Check sheet for the modelled part. Datum: model origin and axes. Units: mm. A direction names the side the tool comes from. Coordinates: 2 decimals unless noted, no trailing zeros. Loops run counter-clockwise (first coordinate to the right, second up) from the corner with the lowest first, then second, coordinate; pieces in that order, holes last. Notation, with made-up numbers: M -37,66 L -31,66 A19 cw -31,80 Z; hole C -11.75,45.5 d5. An arc over 180 degrees is marked long. Write each question's results on one line, items separated by ' | '. Start each with the question number.
from build123d import *

# Parameters (mm, degrees)
SKETCH1_W                      = 96
SKETCH1_H                      = 96
BOSS_EXTRUDE1_DEPTH            = 8
SKETCH2_W                      = 92
SKETCH2_H                      = 92
COMPONENT_PLATFORM_DEPTH       = 6
CABLE_SLOTS_DEPTH              = 6
INNER_CORNER_FILLETS_R         = 3
M3X0_5_TAPPED_HOLE1_AT_2_COUNT = 2
M3X0_5_TAPPED_HOLE1_AT_2_PITCH = 70
M3X0_5_TAPPED_HOLE2_AT_2_COUNT = 2
M3X0_5_TAPPED_HOLE2_AT_2_PITCH = 70
M1_4X0_3_TAPPED_HOLE1_D        = 1.1
M1_4X0_3_TAPPED_HOLE1_DEPTH    = 3.7
M1_4X0_3_TAPPED_HOLE1_TIP      = 0.33047334
SKETCH29_R                     = 12
HDD_EXTRUSION_CUTOUT_DEPTH     = 10
HDD_EXTRUSION_CUTOUT_2_DEPTH   = 10
M3X0_5_TAPPED_HOLE3_D          = 2.5
M3X0_5_TAPPED_HOLE3_DEPTH      = 10
M3X0_5_TAPPED_HOLE3_TIP        = 0.751075774


with BuildPart() as part:
    # Sketch1 → Boss-Extrude1 (new body)
    with BuildSketch(Plane.XY):
        Rectangle(SKETCH1_W, SKETCH1_H)
    extrude(amount=BOSS_EXTRUDE1_DEPTH)

    # Sketch2 → Component Platform (cut)
    with BuildSketch(Plane.XY.offset(8)):
        Rectangle(SKETCH2_W, SKETCH2_H)
    extrude(amount=-COMPONENT_PLATFORM_DEPTH, mode=Mode.SUBTRACT)

    # Sketch3 → Cable Slots (cut, symmetric)
    with BuildSketch(Plane.XY.offset(2)):
        with BuildLine():
            Line((-33.878679656, -25.121320344), (-28.878679656, -20.121320344))
            ThreePointArc((-28.878679656, -20.121320344), (-28.228361402, -19.148050297), (-28, -18))
            Line((-28, -18), (-28, 18))
            ThreePointArc((-28, 18), (-28.228361402, 19.148050297), (-28.878679656, 20.121320344))
            Line((-28.878679656, 20.121320344), (-33.878679656, 25.121320344))
            ThreePointArc((-33.878679656, 25.121320344), (-34.851949703, 25.771638598), (-36, 26))
            Line((-36, 26), (-48, 26))
            Line((-48, 26), (-48, -26))
            Line((-48, -26), (-36, -26))
            ThreePointArc((-36, -26), (-34.851949703, -25.771638598), (-33.878679656, -25.121320344))
        make_face()
        with BuildLine():
            Line((48, -26), (48, 26))
            Line((48, 26), (36, 26))
            ThreePointArc((36, 26), (34.851949703, 25.771638598), (33.878679656, 25.121320344))
            Line((33.878679656, 25.121320344), (28.878679656, 20.121320344))
            ThreePointArc((28.878679656, 20.121320344), (28.228361402, 19.148050297), (28, 18))
            Line((28, 18), (28, -18))
            ThreePointArc((28, -18), (28.228361402, -19.148050297), (28.878679656, -20.121320344))
            Line((28.878679656, -20.121320344), (33.878679656, -25.121320344))
            ThreePointArc((33.878679656, -25.121320344), (34.851949703, -25.771638598), (36, -26))
            Line((36, -26), (48, -26))
        make_face()
    extrude(amount=CABLE_SLOTS_DEPTH, both=True, mode=Mode.SUBTRACT)

    # Inner Corner Fillets
    inner_corner_fillets_edges = [part.edges().sort_by_distance(p)[0] for p in [
        (-46, -46, 5),
        (-46, 46, 5),
        (46, 46, 5),
        (46, -46, 5),
    ]]
    fillet(inner_corner_fillets_edges, radius=INNER_CORNER_FILLETS_R)

    # Sketch14 → M3x0.5 Tapped Hole1 (revolve, cut)
    with BuildSketch(Plane(origin=(48, -35, 5), x_dir=(0, 0, -1), z_dir=(0, 1, 0))):
        Polygon((0, 0), (0, 10.751075774), (1.25, 10), (1.25, 0), align=None)
    m3x0_5_tapped_hole1 = revolve(axis=Axis((54.35, -35, 5), (-1, 0, 0)), mode=Mode.SUBTRACT)

    # M3x0.5 Tapped Hole1 at 2: M3x0.5 Tapped Hole1 ×2
    with Locations(*[(0, i * M3X0_5_TAPPED_HOLE1_AT_2_PITCH, 0) for i in range(1, M3X0_5_TAPPED_HOLE1_AT_2_COUNT)]):
        add(m3x0_5_tapped_hole1, mode=Mode.SUBTRACT)

    # Sketch16 → M3x0.5 Tapped Hole2 (revolve, cut)
    with BuildSketch(Plane(origin=(35, 48, 5), x_dir=(0, 0, 1), z_dir=(1, 0, 0))):
        Polygon((0, 0), (0, 10.751075774), (1.25, 10), (1.25, 0), align=None)
    m3x0_5_tapped_hole2 = revolve(axis=Axis((35, 54.35, 5), (0, -1, 0)), mode=Mode.SUBTRACT)

    # M3x0.5 Tapped Hole2 at 2: M3x0.5 Tapped Hole2 ×2
    with Locations(*[(-i * M3X0_5_TAPPED_HOLE2_AT_2_PITCH, 0, 0) for i in range(1, M3X0_5_TAPPED_HOLE2_AT_2_COUNT)]):
        add(m3x0_5_tapped_hole2, mode=Mode.SUBTRACT)

    # Mirror1: M3x0.5 Tapped Hole1 across plane
    add(m3x0_5_tapped_hole1.mirror(Plane(origin=(0, 0, 0), x_dir=(0, 0, 1), z_dir=(1, 0, 0))), mode=Mode.SUBTRACT)

    # Mirror1 copy 1 sketch → Mirror1 copy 1 (revolve, cut)
    with BuildSketch(Plane(origin=(-48, 35, 5), x_dir=(0, 0, -1), z_dir=(0, 1, 0))):
        Polygon((0, 0), (0, -10.751075774), (1.25, -10), (1.25, 0), align=None)
    revolve(axis=Axis((-54.35, 35, 5), (-1, 0, 0)), mode=Mode.SUBTRACT)

    # Mirror2: M3x0.5 Tapped Hole2 across plane
    add(m3x0_5_tapped_hole2.mirror(Plane(origin=(0, 0, 0), x_dir=(0, 0, 1), z_dir=(0, -1, 0))), mode=Mode.SUBTRACT)

    # Mirror2 copy 1 sketch → Mirror2 copy 1 (revolve, cut)
    with BuildSketch(Plane(origin=(-35, -48, 5), x_dir=(0, 0, 1), z_dir=(1, 0, 0))):
        Polygon((0, 0), (0, -10.751075774), (1.25, -10), (1.25, 0), align=None)
    revolve(axis=Axis((-35, -54.35, 5), (0, -1, 0)), mode=Mode.SUBTRACT)

    # M1.4x0.3 Tapped Hole1
    with Locations(Plane.XY.offset(2)):
        with Locations((-19.31998517, -29.75), (24.78001483, -32.85), (-22.91998517, 32.85)):
            Hole(M1_4X0_3_TAPPED_HOLE1_D / 2, depth=M1_4X0_3_TAPPED_HOLE1_DEPTH)
            with Locations((0, 0, -(M1_4X0_3_TAPPED_HOLE1_DEPTH + M1_4X0_3_TAPPED_HOLE1_TIP / 2))):  # 118° drill point
                Cone(0, M1_4X0_3_TAPPED_HOLE1_D / 2, M1_4X0_3_TAPPED_HOLE1_TIP, mode=Mode.SUBTRACT)

    # Sketch29 → HDD Extrusion Cutout (cut)
    with BuildSketch(Plane(origin=(0, 0, 0), x_dir=(-1, 0, 0), z_dir=(0, 0, -1))):
        with Locations((-0.08192631, -8.74785827)):
            Circle(SKETCH29_R)
    extrude(amount=-HDD_EXTRUSION_CUTOUT_DEPTH, mode=Mode.SUBTRACT)

    # Sketch9 → HDD Extrusion Cutout 2 (cut)
    with BuildSketch(Plane.XY.offset(2)):
        with BuildLine():
            Line((25, 31), (25, 15))
            ThreePointArc((25, 15), (24.414213562, 13.585786438), (23, 13))
            Line((23, 13), (17, 13))
            ThreePointArc((17, 13), (8.514718626, 16.514718626), (5, 25))
            Line((5, 25), (5, 31))
            ThreePointArc((5, 31), (5.585786438, 32.414213562), (7, 33))
            Line((7, 33), (23, 33))
            ThreePointArc((23, 33), (24.414213562, 32.414213562), (25, 31))
        make_face()
    extrude(amount=-HDD_EXTRUSION_CUTOUT_2_DEPTH, mode=Mode.SUBTRACT)

    # M3x0.5 Tapped Hole3
    with Locations(Plane.XY.offset(2)):
        with Locations((-31.790998517, -39.06), (31.29001483, -39.06), (31.29001483, 38.94), (-31.790998517, 38.94)):
            Hole(M3X0_5_TAPPED_HOLE3_D / 2, depth=M3X0_5_TAPPED_HOLE3_DEPTH)
            with Locations((0, 0, -(M3X0_5_TAPPED_HOLE3_DEPTH + M3X0_5_TAPPED_HOLE3_TIP / 2))):  # 118° drill point
                Cone(0, M3X0_5_TAPPED_HOLE3_D / 2, M3X0_5_TAPPED_HOLE3_TIP, mode=Mode.SUBTRACT)


solid = part.part
1) Thickness scan on probe 1 along Y at (x, z) = (47.25, 5); probe 2 along Z at (x, y) = (35, -46.45); probe 3 along Y at (x, z) = (-33.5, 2.5). Record the ranges inside material, lowest first.
2) Section check A-A (x = 38). Enter the section's corners in (y, z).
3) Section check B-B (y = -35). Enter the section's corners in (x, z).
4) Section check D-D (z = 5). Give the number of separate pieces and of enclosed holes in the cut face, then the cut area to 3 significant figures.
5) Gauge pin test, flat ends, axial feed: P1, Ø6, axis at x = -23, y = 32, coming from the +Z side; P2, Ø2, axis at y = 35, z = 5, coming from the +X side. Record the tip position at first contact, or that the pin passes through.
6) Release check for a two-part mould opening along Y. For faces 1 (the flat face through (-48, -37, 4)), 2 (the cylindrical face through (-30.54, 38.99, 0.99)) record: +Y half, -Y half, draft (parallel to the pull), parting line (faces both ways), or undercut.
7) Set-up check for faces 3 (the flat face through (46, 34, 4)), 4 (the cylindrical face through (8.61, 16.42, 1.01)), 5 (the flat face through (-31.344, 22.586, 0.986)): record each of +Z, -Z, +X, -X, +Y, -Y from which the full face is reachable in a straight line by a thin tool's end or side.
8) Section check C-C (y = -13.5). Enter the section's corners in (x, z), then the cut area to 3 significant figures.
Return value:
1) probe 1: y = -48 to -36.25, -33.75 to -26, 26 to 33.75, 36.25 to 48 | probe 2: z = 0 to 3.75, 6.25 to 8 | probe 3: y = -48 to -46, 46 to 48
2) outline: M -48,0 L -26,0 L -26,2 L -46,2 L -46,8 L -48,8 Z; M 26,0 L 48,0 L 48,8 L 46,8 L 46,2 L 26,2 Z
3) outline: M -48,0 L 48,0 L 48,3.75 L 46,3.75 L 46,2 L -46,2 L -46,3.75 L -48,3.75 Z; M -48,6.25 L -46,6.25 L -46,8 L -48,8 Z; M 46,6.25 L 48,6.25 L 48,8 L 46,8 Z
4) separate pieces: 10 | enclosed holes: 0 | area: 512 mm2
5) P1: stops at z = 2 | P2: passes through
6) face 1: draft | face 2: undercut
7) face 3: +Z | face 4: +Z, -Z | face 5: +Z, -Z, -X
8) outline: M -28,0 L -10.94,0 L -10.94,2 L -28,2 Z; M 11.1,0 L 28,0 L 28,2 L 11.1,2 Z | area: 67.9 mm2
